The drawing under review shows one solid part. Ordinate dimensions are in mm from its lowest x, y, z. A direction names the side the tool comes from. Give positions to 0.01 mm unless a question says otherwise; leave off trailing zeros. Order: outer loops, then holes, each group sorted by start corner. A loop starts at its lowest first (then second) coordinate and runs counter-clockwise, first axis right, second up. Notation, with made-up numbers: (70.25, -30.5) - (91.25, -30.5) arc R32 ccw to (91.25, 5.5) - close; hole circle Ø9 at (79, -29.75). An arc over 180 degrees is marked (long way). Use CSV: the item, a comma, the result in double quotes.
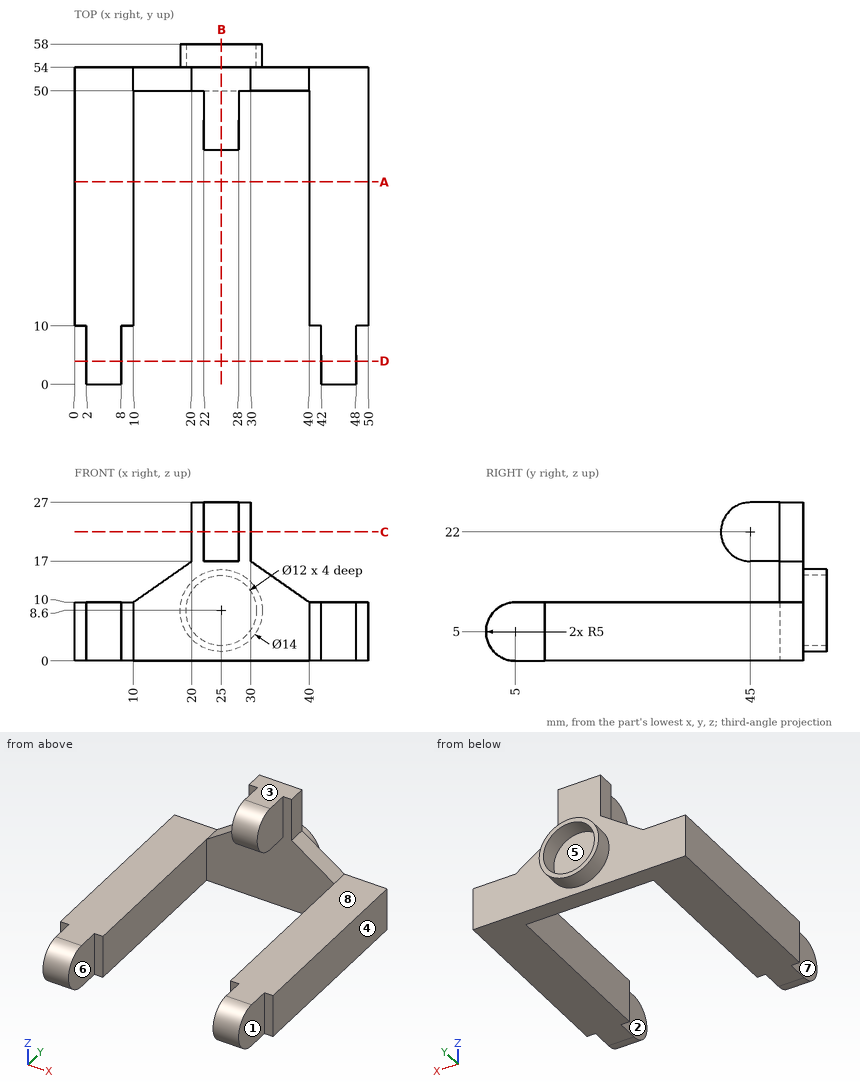
Item 1: Tool access review of the marked faces 1, 2, 3, 4 and 5: name each direction out of +Z, -Z, +X, -X, +Y, -Y from which nothing blocks a thin tool from reaching the whole face with its end or side.
Results list:
face 1,"+Z, -Z, +X, -Y"
face 2,"+Z, -Z, -Y"
face 3,"+Z, +X, -X, +Y, -Y"
face 4,"+Z, -Z, +X, +Y, -Y"
face 5,"+Y"
Item 2: Take a section at D-D, the plane y = 4. Give the boundary of the cut face in (x, z), and give its area (3 significant figures).
Results list:
outline,"(2, 0.1) - (8, 0.1) - (8, 9.9) - (2, 9.9) - close; (42, 0.1) - (48, 0.1) - (48, 9.9) - (42, 9.9) - close"
area,"118 mm2"
Item 3: Take a section at A-A, the plane y = 34.5. Give the boundary of the cut face in (x, z).
Results list:
outline,"(0, 0) - (10, 0) - (10, 10) - (0, 10) - close; (40, 0) - (50, 0) - (50, 10) - (40, 10) - close"
Item 4: Clearance check with flat-ended pins moving along their axes: pin 1 (5 mm diameter, centred on y = 3.5, z = 5.5, fed in from +X); pin 2 (1 mm diameter, centred on x = 9, z = 6, fed in from -Y); pin 3 (6 mm diameter, centred on x = 24.5, z = 7, fed in from +Y). State where each tip first meets the part, or that it passes through.
Results list:
pin 1,"stops at x = 48"
pin 2,"stops at y = 10"
pin 3,"stops at y = 54"
Item 5: Mouldability with a two-part tool opening along X and no side actions: class the marked faces 6, 7 and 8 as pulls with the +X half, pulls with the -X half, needs draft (parallel to the pull), parting line crosses it, or undercut.
Results list:
face 6,"undercut"
face 7,"pulls with the -X half"
face 8,"needs draft"
Item 6: Wall thickness on L1, parallel to X at y = 55.35, z = 8.6; L2, parallel to X at y = 16, z = 2.75; L3, parallel to Z at x = 25, y = 55.35: over which ranges is each line inside the solid? List them lowest first.
Results list:
L1,"x = 18 to 19, 31 to 32"
L2,"x = 0 to 10, 40 to 50"
L3,"z = 1.6 to 2.6, 14.6 to 15.6"
Item 7: Take a section at C-C, the plane z = 22. Give the boundary of the cut face in (x, y), and give its area (3 significant figures).
Results list:
outline,"(20, 50) - (22, 50) - (22, 40) - (28, 40) - (28, 50) - (30, 50) - (30, 54) - (20, 54) - close"
area,"100 mm2"
Item 8: Take a section at B-B, the plane x = 25. Give the boundary of the cut face in (y, z).
Results list:
outline,"(45, 17) - (50, 17) - (50, 0) - (54, 0) - (54, 1.6) - (58, 1.6) - (58, 2.6) - (54, 2.6) - (54, 14.6) - (58, 14.6) - (58, 15.6) - (54, 15.6) - (54, 27) - (45, 27) arc R5 ccw to start"
